Source: CAD feature listing. Evaluate the final solid. Frame: model axes, mm. A direction names the side the tool comes from. Round coordinates to 2 decimals unless told otherwise and drop trailing zeros. Order: outer loops, then holes, each group sorted by start corner. A loop starts at its lowest first (then second) coordinate and runs counter-clockwise, first axis right, second up. Notation, with made-up numbers: (22.5, -39.5) - (37.5, -39.5) arc R20 cw to (37.5, -16.5) - close; hole circle Ø1 at (73, -4). An arc over 180 degrees is marked (long way). Return JSON: item names as keys, results as strings. Group by question number.
1) Mould query, pull axis Z, two halves, no side actions, for faces 1 (the flat face through (4, 0, -4)), 2 (the flat face through (-1, 20.5, 19)), 3 (the cylindrical face through (0.33, 1.564, -7.493)). Classes: pulls with the +Z half, pulls with the -Z half, needs draft (parallel to the pull), parting line crosses it, or undercut.
2) Section B-B, the plane y = 8.25. Return loops of the section in (x, z), plus the area to 3 significant figures.
3) Ray query, line 1 (X direction, y = 14.5, z = 6.5); line 2 (Z direction, x = -2, y = 18); line 3 (Z direction, x = -11, y = 17.5). Return the intervals inside material, ascending. Write a range as from..to.
4) Contact query for flat-ended pins moving along their axis: P1, Ø1.5, axis at x = -11.5, z = -17.5, coming from the +Y side; P2, Ø12, axis at x = -14.5, z = 9, coming from the -Y side; P3, Ø5, axis at y = 14.5, z = 9, coming from the +X side; P4, Ø6, axis at x = -15.5, y = 5, coming from the -Z side. Output: stop coordinate, or through.
5) Section A-A, the plane z = 0. Return loops of the section in (x, y), plus the area to 3 significant figures.
6) Access query for faces 4 (the flat face through (4, 12, -4)), 5 (the flat face through (0, 6, 6.4)), 6 (the conical face through (0.206, 0.358, -5.138)). Directions: +Z, -Z, +X, -X, +Y, -Y. A direction counts if a zero-diameter tool reaches every point of the face in a straight line with its end or side. Return the directions, or none.
```python
from build123d import *

# Parameters (mm, degrees)
SKETCH_1_R             = 7.5
EXTRUDE_1_DEPTH        = 12
CUT_EXTRUDE_1_DEPTH    = 36.334119621
CHAMFER_1_SIZE         = 0.5
HOLE_WIZARD_1_D        = 4.5
HOLE_WIZARD_1_DEPTH    = 1.5
HOLE_WIZARD_M3_1_D     = 2.5
HOLE_WIZARD_M3_1_DEPTH = 3.248924226
HOLE_WIZARD_M3_1_TIP   = 0.751075774


with BuildPart() as part:
    # 草图1 → 凸台-拉伸1 (new body)
    with BuildSketch(Plane(origin=(0, 0, 0), x_dir=(1, 0, 0), z_dir=(0, 1, 0))):
        with Locations(Location((0, 0, 0), (0, 0, 270))):
            Circle(SKETCH_1_R)
    extrude(amount=EXTRUDE_1_DEPTH)

    # 草图2 → 旋转1 (revolve)
    with BuildSketch(Plane.XY, mode=Mode.PRIVATE) as revolve_1_sk:
        with BuildLine():
            Line((2.982229812, 4.310656936), (5.810656936, 1.482229812))
            Line((5.810656936, 1.482229812), (19.383203961, 15.054776836))
            ThreePointArc((19.383203961, 15.054776836), (22.474873734, 20.974873734), (16.554776836, 17.883203961))
            Line((16.554776836, 17.883203961), (2.982229812, 4.310656936))
        make_face()
    revolve(revolve_1_sk.sketch.rotate(Axis((0, 0, 0), (0, 1, 0)), 270), axis=Axis((0, 0, 0), (0, 1, 0)))

    # 草图3 → 切除-拉伸1 (cut, through all)
    with BuildSketch(Plane(origin=(0, 12, 0), x_dir=(1, 0, 0), z_dir=(0, 1, 0))):
        with BuildLine():
            Line((-1.5, -4.769696007), (-1.5, -6.4))
            Line((-1.5, -6.4), (1.5, -6.4))
            Line((1.5, -6.4), (1.5, -4.769696007))
            ThreePointArc((1.5, -4.769696007), (0, 5), (-1.5, -4.769696007))
        make_face()
    extrude(amount=-CUT_EXTRUDE_1_DEPTH, mode=Mode.SUBTRACT)

    # 倒角1
    chamfer_1_edges = [part.edges().sort_by_distance(p)[0] for p in [
        (0, 0, -5),
        (0, 12, -5),
    ]]
    chamfer(chamfer_1_edges, length=CHAMFER_1_SIZE)

    # 孔1
    with Locations(Plane(origin=(0, 22, 20), x_dir=(0, 0, 1), z_dir=(0, 1, 0))):
        with Locations((0, 0)):
            Hole(HOLE_WIZARD_1_D / 2, depth=HOLE_WIZARD_1_DEPTH)

    # M3 螺纹孔1
    with Locations(Plane(origin=(0, 20.5, 0), x_dir=(1, 0, 0), z_dir=(0, 1, 0))):
        with Locations((0, -20), (0, 0)):
            Hole(HOLE_WIZARD_M3_1_D / 2, depth=HOLE_WIZARD_M3_1_DEPTH)
            with Locations((0, 0, -(HOLE_WIZARD_M3_1_DEPTH + HOLE_WIZARD_M3_1_TIP / 2))):  # 118° drill point
                Cone(0, HOLE_WIZARD_M3_1_D / 2, HOLE_WIZARD_M3_1_TIP, mode=Mode.SUBTRACT)


solid = part.part
```
Geometry check:
{
 "1": {"face 1": "needs draft", "face 2": "undercut", "face 3": "parting line crosses it"},
 "2": {"outline": "circle Ø25.16 at (0, 0); hole (-1.5, 4.77) arc R5 ccw (long way) to (1.5, 4.77) - (1.5, 6.4) - (-1.5, 6.4) - close", "area": "414 mm2"},
 "3": {"line 1": "-17.67..-11.46, 11.46..17.67", "line 2": "-23.38..-16.41, 16.41..23.38", "line 3": "-20.6..-11.85, 11.85..20.6"},
 "4": {"P1": "y = 21.99", "P2": "y = 6.74", "P3": "x = 21.63", "P4": "through"},
 "5": {"outline": "(-19.38, 15.05) - (-7.5, 3.17) - (-7.5, 0) - (-5.5, 0) - (-5, 0.5) - (-5, 11.5) - (-5.5, 12) - (-7.5, 12) - (-7.5, 8.83) - (-16.55, 17.88) arc R3.5 ccw (long way) to start; (5, 0.5) - (5.5, 0) - (7.5, 0) - (7.5, 3.17) - (19.38, 15.05) arc R3.5 ccw (long way) to (16.55, 17.88) - (7.5, 8.83) - (7.5, 12) - (5.5, 12) - (5, 11.5) - close", "area": "251 mm2"},
 "6": {"face 4": "+Y", "face 5": "+Y, -Y", "face 6": "-Y"}
}
